Design review of the part shown in the three views and the two pictorial views. Dimensions are in mm from the part's minimum x, y and z. Coordinates: 2 decimals unless noted, no trailing zeros. Write each loop counter-clockwise with the first axis right and the second up, starting at its lowest first coordinate (ties: lowest second). Pieces come first, ordered by that corner, then holes. Notation, with made-up numbers: M 32.5,-9.75 L 60.5,-9.75 A26 ccw 60.5,19.25 Z; hole C -3,-40 d3. An arc over 180 degrees is marked long. Answer as a JSON object with one key per item and string values.
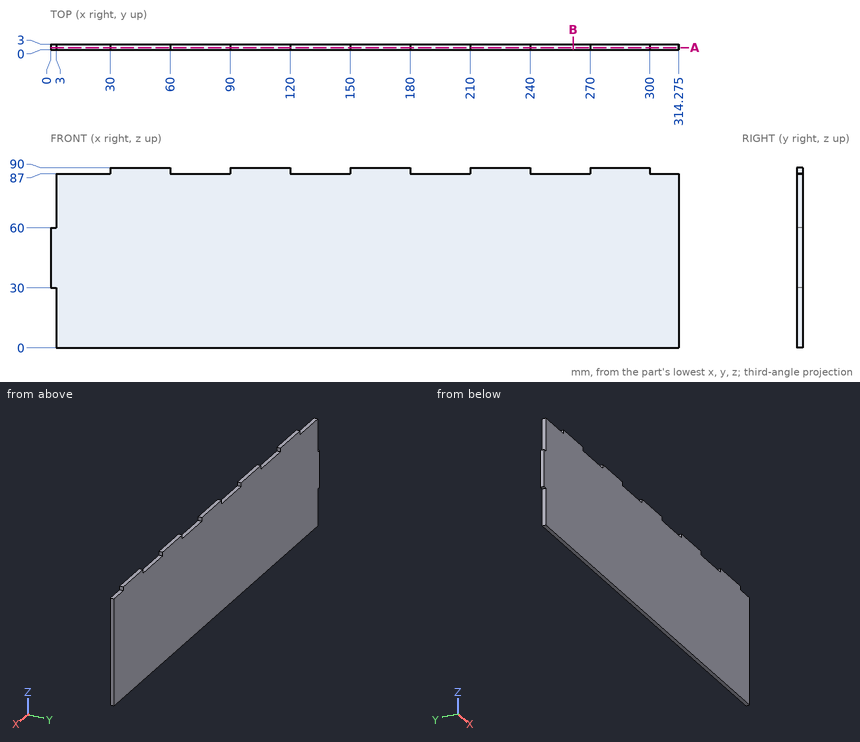
(1) Add section B-B on x = 261.5. Give the boundary of the cut face in (y, z).
Results list:
{"outline": "M 0,0 L 3,0 L 3,87 L 0,87 Z"}
(2) For pin 1 Ø1.5 at (x, y) = (306, 2) entering from +Z; pin 2 Ø1.5 at (y, z) = (1, 88.5) entering from +X; pin 3 Ø1.5 at (y, z) = (1.5, 74.5) entering from -X, all flat-tipped, find the tip position at first contact; note any pin that passes through.
Results list:
{"pin 1": "z = 87", "pin 2": "x = 300", "pin 3": "x = 3"}
(3) Wall thickness on line 1 along Z through (x, y) = (15.5, 2.25); line 2 along X through (y, z) = (1.65, 23.5) (3 decimals): over which ranges is each line inside the solid? List them lowest first. Write a range as from..to.
Results list:
{"line 1": "0..87", "line 2": "3..314.275"}
(4) Add section A-A on y = 1.2. Give the boundary of the cut face in (x, z) (3 decimals).
Results list:
{"outline": "M 0,30 L 3,30 L 3,0 L 314.275,0 L 314.275,87 L 300,87 L 300,90 L 270,90 L 270,87 L 240,87 L 240,90 L 210,90 L 210,87 L 180,87 L 180,90 L 150,90 L 150,87 L 120,87 L 120,90 L 90,90 L 90,87 L 60,87 L 60,90 L 30,90 L 30,87 L 3,87 L 3,60 L 0,60 Z"}
